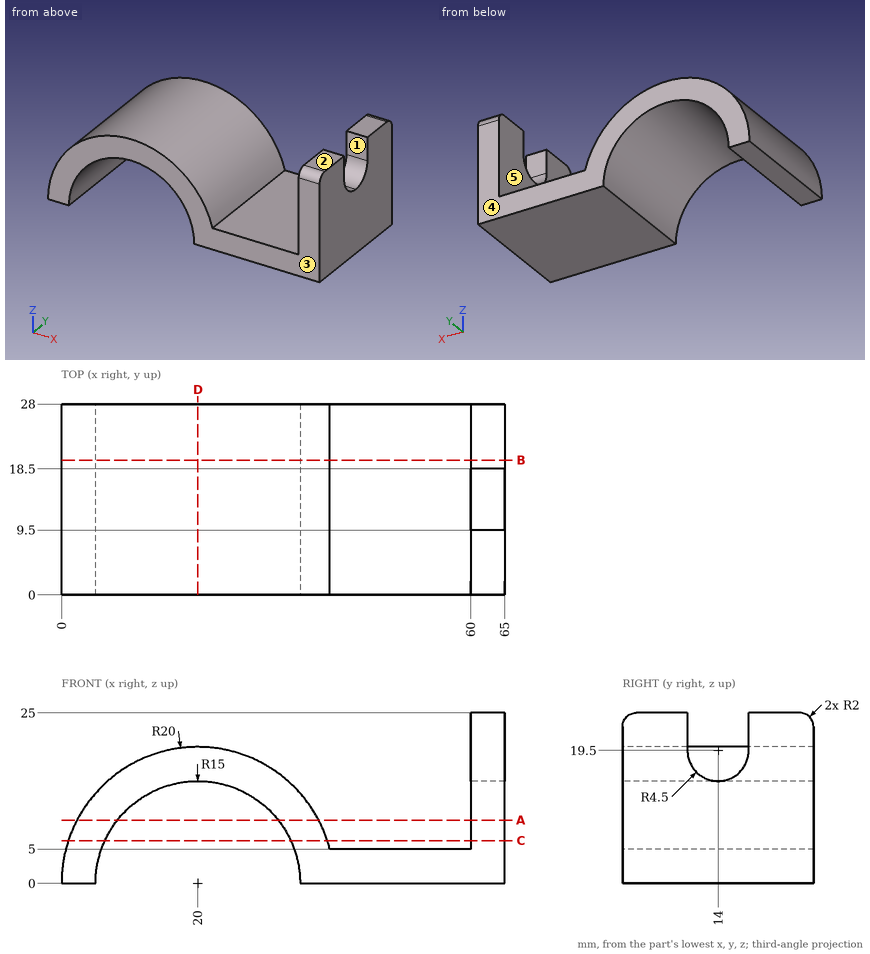
Can you work these out from the drawing? Everything is in mm from the part's minimum corner. A direction names the side the tool comes from. Give positions to 0.01 mm unless a question says otherwise; leave off trailing zeros. Loops run counter-clockwise (first coordinate to the right, second up) from the corner with the lowest first, then second, coordinate; pieces in that order, holes last. Notation, with made-up numbers: (-39.75, -20.5) - (14.25, -20.5) arc R18 ccw to (14.25, -2.5) - close; hole circle Ø1 at (81, 28). An arc over 180 degrees is marked (long way). Answer as a JSON object with one key per item and string values.
Q1. If I drill on L1, parallel to X at y = 25, z = 12.5; L2, parallel to X at y = 13.25, z = 9; L3, parallel to Z at x = 46, y = 21.5, over which ranges is the centre line in solid material (lowest first)?
Geometry says:
{"L1": "4.39 to 11.71, 28.29 to 35.61, 60 to 65", "L2": "2.14 to 8, 32 to 37.86, 60 to 65", "L3": "0 to 5"}
Q2. Imagine slicing it at B-B on y = 19.75. Write out the boundary of the cut face in (x, z), plus the area to 3 significant figures.
Geometry says:
{"outline": "(0, 0) - (5, 0) arc R15 cw to (35, 0) - (65, 0) - (65, 25) - (60, 25) - (60, 5) - (39.36, 5) arc R20 ccw to start", "area": "501 mm²"}
Q3. Imagine slicing it at D-D on x = 20. Write out the boundary of the cut face in (y, z), plus the area to 3 significant figures.
Geometry says:
{"outline": "(0, 15) - (28, 15) - (28, 20) - (0, 20) - close", "area": "140 mm²"}
Q4. Imagine slicing it at A-A on z = 9.25. Write out the boundary of the cut face in (x, y).
Geometry says:
{"outline": "(2.27, 0) - (8.19, 0) - (8.19, 28) - (2.27, 28) - close; (31.81, 0) - (37.73, 0) - (37.73, 28) - (31.81, 28) - close; (60, 0) - (65, 0) - (65, 28) - (60, 28) - close"}
Q5. Will these pins go through, and if not, where does the flat tip stop? P1, Ø6, axis at x = 36.5, y = 23, coming from the +Z side; P2, Ø1.5, axis at y = 24, z = 15.5, coming from the -X side; P3, Ø16.5, axis at x = 48, y = 8.5, coming from the +Z side.
Geometry says:
{"P1": "z = 14.76", "P2": "x = 6.49", "P3": "z = 5"}
Q6. If we mould it in two halves opening along Y, with no side actions, what happens to the marked faces 1, 2 and 3? For each: pulls with the +Y half, pulls with the -Y half, needs draft (parallel to the pull), parting line crosses it, or undercut.
Geometry says:
{"face 1": "undercut", "face 2": "needs draft", "face 3": "pulls with the -Y half"}
Q7. Which directions (+Z, -Z, +X, -X, +Y, -Y) give clear straight access to the entire face, cutting with the end or side of a thin tool? Please do the marked faces 4 and 5.
Geometry says:
{"face 4": "+Z, -Z, +X, -X, +Y", "face 5": "+Z, +Y, -Y"}
Q8. Imagine slicing it at C-C on z = 6.25. Write out the boundary of the cut face in (x, y).
Geometry says:
{"outline": "(1, 0) - (6.36, 0) - (6.36, 28) - (1, 28) - close; (33.64, 0) - (39, 0) - (39, 28) - (33.64, 28) - close; (60, 0) - (65, 0) - (65, 28) - (60, 28) - close"}
